Build history of the part. All positions in model axes, mm. A direction names the side the tool comes from. Coordinates: 2 decimals unless noted, no trailing zeros. Loops run counter-clockwise (first coordinate to the right, second up) from the corner with the lowest first, then second, coordinate; pieces in that order, holes last. Notation, with made-up numbers: (-21, 53) - (-3, 53) arc R5 ccw to (-3, 59) - close; hole circle Ø10 at (-26, 5). An arc over 180 degrees is marked (long way). One line per item, written item: value.
Autodesk Inventor part; units mm, degrees
ref_plane "YZ Plane" through (0, 0, 0) normal (1, 0, 0) x (0, 1, 0)
ref_plane "XZ Plane" through (0, 0, 0) normal (0, 1, 0) x (-1, 0, 0)
ref_plane "XY Plane" through (0, 0, 0) normal (0, 0, 1) x (1, 0, 0)
sketch "Sketch1" plane through (0, 0, 0) normal (1, 0, 0) x (0, 1, 0)
  line L0 (12.5, 55) -> (-12.5, 55)
  line L1 (-12.5, 55) -> (-12.5, -55)
  line L2 (-12.5, -55) -> (12.5, -55)
  line L3 (12.5, -55) -> (12.5, 55)
  arc A0 (12.5, 55) -> (-12.5, 55) centre (0, 55) ccw
  arc A1 (-12.5, -55) -> (12.5, -55) centre (0, -55) ccw
  circle A2 centre (0, 55) radius 1.65
  circle A3 centre (0, 55) radius 3.75
  circle A4 centre (0, 55) radius 8.25
  line L4 (4, 55) -> (-4, 55)
  line L5 (-4, 55) -> (-4, 27.25)
  line L6 (-4, 27.25) -> (4, 27.25)
  line L7 (4, 27.25) -> (4, 55)
  circle A5 centre (0, 31) radius 1.65
  circle A6 centre (0, 36) radius 1.65
  line L8 (1.65, 36) -> (1.65, 31)
  line L9 (-1.65, 36) -> (-1.65, 31)
  line L10 (12.5, 0) -> (-12.5, 0) construction
  circle A7 centre (0, -55) radius 1.65
  circle A8 centre (0, -55) radius 3.75
  circle A9 centre (0, -55) radius 8.25
  line L11 (-4, -55) -> (-4, -27.25)
  line L12 (-4, -27.25) -> (4, -27.25)
  line L13 (4, -27.25) -> (4, -55)
  circle A10 centre (0, -31) radius 1.65
  circle A11 centre (0, -36) radius 1.65
  line L14 (1.65, -36) -> (1.65, -31)
  line L15 (-1.65, -36) -> (-1.65, -31)
  line L16 (4.5, 25) -> (-4.5, 25)
  line L17 (-4.5, 25) -> (-4.5, -25)
  line L18 (-4.5, -25) -> (4.5, -25)
  line L19 (4.5, -25) -> (4.5, 25)
  line L20 (4.5, 25) -> (-4.5, -25) construction
  line L21 (-4.5, 25) -> (4.5, -25) construction
  arc A12 (-4.5, 25) -> (4.5, 25) centre (0, 33.9303) ccw
  arc A13 (4.5, -25) -> (-4.5, -25) centre (0, -33.9303) ccw
  point P0 (0, 0)
  point P1 (0, 55)
  point P2 (-4, -47.7846)
  point P3 (4, -47.7846)
  point P4 (4, 47.7846)
  point P5 (-4, 47.7846)
  point P6 (0, 0)
  point P7 (3.75, 55)
  point P8 (-3.75, 55)
  dimension "d0" = 110
  dimension "d1" = 55
  dimension "d2" = 12.5
  dimension "d3" = 25
  dimension "d4" = 3.3
  dimension "d5" = 7.5
  dimension "d6" = 16.5
  dimension "d7" = 8
  dimension "d8" = 4
  dimension "d10" = 36
  dimension "d11" = 3.3
  dimension "d12" = 24
  dimension "d13" = 4
  dimension "d14" = 3.3
  dimension "d15" = 5
  dimension "d16" = 4
  dimension "d34" = 50
  dimension "d35" = 8
  dimension "d36" = 8
  dimension "d37" = 10
  dimension "d38" = 10
extrude "Extrusion1" add sketch "Sketch1" along normal blind 6 contours L3 L2 A9 L13 L12 L11 L1 L0 A4 L5 L6 L7 | L0 A4 A0 | A1 L2 A9 | A12 L16 | L18 A13
extrude "Extrusion2" add sketch "Sketch1" against normal blind 2 contours L3 L2 A9 L13 L12 L11 L1 L0 A4 L5 L6 L7 | L0 A4 A0 | A4 L7 L0 | L0 A3 A4 | A1 L2 A9 | L7 A4 L5 L0 A3 | L0 L5 A4 | L7 L6 L5 A4 | A9 L2 A8 | L2 L13 A9 | A3 L0 A2 | L0 A2 A3 | L2 A8 L11 A9 L13 | A9 L11 L12 L13 | A9 L11 L2 | A8 L2 A7 | L2 A7 A8 | A12 L16 | L18 A13
extrude "Extrusion3" add sketch "Sketch1" along normal blind 1 contours A3 L0 A2 | L0 A2 A3 | A8 L2 A7 | L2 A7 A8
fillet "Fillet1" radius 4 4 edges at (3, -4, 27.25) (3, 4, 27.25) (3, -4, -27.25) (3, 4, -27.25)
fillet "Fillet2" radius 8 4 edges at (3, -4, -47.7846) (3, 4, -47.7846) (3, -4, 47.7846) (3, 4, 47.7846)
fillet "Fillet3" radius 2 8 edges at (6, 0, 67.5) (6, -12.5, 0) (6, 0, -67.5) (6, 12.5, 0) (-2, 0, -67.5) (-2, -12.5, 0) (-2, 0, 67.5) (-2, 12.5, 0)
equation "\"d0\" = FEMUR_LENGTH"
equation "\"d3\" = FEMUR_WIDTH"
equation "\"d4\" = HornScrewDiameter"
equation "\"d5\" = HornCentreDiameter"
equation "\"d6\" = HornDiameter"
equation "\"d7\" = HornWidth"
equation "\"d8\" = 0.5 * HornWidth"
equation "\"d10\" = HornLength"
equation "\"d11\" = HornScrewDiameter"
equation "\"d13\" = 0.5 * HornWidth"
equation "\"d14\" = HornScrewDiameter"
equation "\"d15\" = HornScrewLen"
equation "\"d16\" = 0.5 * HornWidth"
equation "\"d17\" = HornHeight"
equation "\"d19\" = FEMUR_HEIGHT - HornHeight"
equation "\"d21\" = HornCentreHeight"
equation "\"d23\" = 0.5 * HornWidth"
equation "\"d24\" = HornFillet"
equation "\"d25\" = PART_FILLET"
properties part number "FemurHornSide"
Item 1: Drop flat-ended pins along their axis: P1, Ø2.5, axis at y = 0, z = -55, coming from the +X side; P2, Ø1.6, axis at x = -1, z = -33, coming from the +Y side; P3, Ø2, axis at y = 1, z = 56, coming from the +X side; P4, Ø1, axis at x = 3.5, y = -6.5, coming from the -Z side. Give the stop position or say it passes through.
Check result:
P1: passes through
P2: stops at y = 12.49
P3: stops at x = 1
P4: stops at z = -65.97
Item 2: Tool access for faces 3 (the face through (-2, -5, 1)), 4 (the face through (2, 4.5, 0)), 5 (the face through (3.042, -2.859, 28.453)): list every direction of +Z, -Z, +X, -X, +Y, -Y with a clear straight run to the whole face (end or side of a thin tool).
Check result:
face 3: +Z, -Z, -X, +Y, -Y
face 4: +X, -X
face 5: +X
Item 3: Probe probe 1 along Z at (x, y) = (4.5, 7.5); probe 2 along Y at (x, z) = (2.7, 55); probe 3 along Z at (x, y) = (-1, -0.5). List the from-to ranges inside material, lowest first. Write a range as from..to.
Check result:
probe 1: z = -64.92..-58.44, -51.56..51.56, 58.44..64.92
probe 2: y = -12.5..-8.25, 8.25..12.5
probe 3: z = -67.22..-56.57, -53.43..-37.57, -29.43..-23.94, 23.94..29.43, 37.57..53.43, 56.57..67.22
Item 4: Pull direction Z, two halves, no side cores. Call faces 1 (the face through (3, -4, -38)), 2 (the face through (2, -12.5, 1)): released by +Z, released by -Z, zero draft, split by the parting line, or undercut.
Check result:
face 1: undercut
face 2: zero draft
Item 5: Cut at A-A, the plane z = 12.5. Write the cut outline in (x, y), then the cut area to 3 significant figures.
Check result:
outline: (-2, -10.5) arc R2 ccw to (0, -12.5) - (4, -12.5) arc R2 ccw to (6, -10.5) - (6, -4.5) - (-2, -4.5) - close; (-2, 4.5) - (6, 4.5) - (6, 10.5) arc R2 ccw to (4, 12.5) - (0, 12.5) arc R2 ccw to (-2, 10.5) - close
area: 125 mm^2
Item 6: Cut at B-B, the plane x = 2.75. Give the number of separate pieces and of enclosed holes in the cut face, then the cut area to 3 significant figures.
Check result:
separate pieces: 1
enclosed holes: 3
area: 2,070 mm^2
